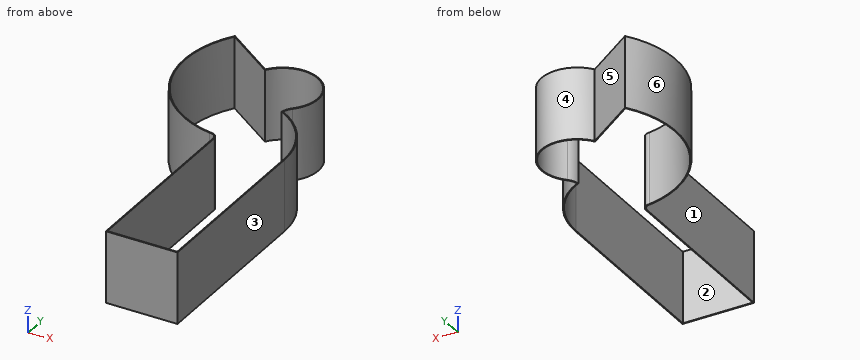
Autodesk Inventor part; units mm, degrees
ref_plane "YZ Plane" through (0, 0, 0) normal (1, 0, 0) x (0, 1, 0)
ref_plane "XZ Plane" through (0, 0, 0) normal (0, 1, 0) x (-1, 0, 0)
ref_plane "XY Plane" through (0, 0, 0) normal (0, 0, 1) x (1, 0, 0)
sketch "Sketch1" plane through (0, 0, 0) normal (0, 0, 1) x (1, 0, 0)
  circle A0 centre (330.2, 1028.7) radius 101.6
  arc A1 (101.3289, 1188.9573) -> (284.1769, 753.1166) centre (330.2, 1028.7) ccw
  circle A2 centre (285.75, 734.1316) radius 19.05
  line L0 (330.2, 1028.7) -> (431.8, 1028.7) construction
  line L1 (0, 1023.3941) -> (50.8, 1023.3941)
  line L2 (50.8, 1023.3941) -> (50.8, 972.5941)
  line L3 (50.8, 972.5941) -> (0, 972.5941)
  line L4 (0, 972.5941) -> (0, 1023.3941)
  line L5 (0, 0) -> (685.8, 0) construction
  line L6 (685.8, 1498.6) -> (0, 1498.6) construction
  line L7 (0, 1498.6) -> (0, 0) construction
  line L8 (304.8, 734.1316) -> (304.8, 213.868)
  line L9 (101.3289, 1188.9573) -> (318.1431, 1498.6) construction
  line L10 (101.3289, 1188.9573) -> (685.8, 1188.9573) construction
  arc A3 (508, 734.1316) -> (260.3446, 954.9248) centre (285.75, 734.1316) ccw
  line L11 (508, 734.1316) -> (508, 213.868)
  line L12 (685.8, 1188.9573) -> (685.8, 0) construction
  line L13 (685.8, 228.9727) -> (685.8, 178.1727)
  line L14 (101.3289, 1188.9573) -> (246.9742, 1086.9754)
  line L15 (304.8, 213.868) -> (508, 213.868)
  arc A4 (401.1312, 955.9585) -> (387.7592, 931.5884) centre (434.38, 921.8609) ccw
  dimension "d0" = 203.2
  dimension "d1" = 279.4
  dimension "d3" = 50.8
  dimension "d4" = 1498.6
  dimension "d5" = 685.8
  dimension "d6" = 38.1
  dimension "d9" = 55
  dimension "d10" = 1028.7
  dimension "d14" = 213.868
  dimension "d20" = 304.8
  dimension "d21" = 177.8
extrude "Extrusion1" add sketch "Sketch1" along normal blind 203.2 contours A0 A3 | A0 A3 L11 L15 L8 A2 A1 L14 | A4 A3 A0 | A3 A0
shell "Shell1" thickness 2.54 removed faces 2 at (372.5333, 560.7104, 0) at (440.2667, 387.2892, 203.2)
properties part number "SketchProfile"
Input: part model. Units: mm. Frame: model coordinates. Face numbers are marked on the shaded views. A direction names the side the tool comes from. Give positions to 0.01 mm unless a question says otherwise; leave off trailing zeros. Order: outer loops, then holes, each group sorted by start corner. A loop starts at its lowest first (then second) coordinate and runs counter-clockwise, first axis right, second up. Notation, with made-up numbers: (-29.75, 12) - (-7.75, 12) arc R26 ccw to (-7.75, 27) - close; hole circle Ø11 at (-29, 88). An arc over 180 degrees is marked (long way). Put each result on its own line as item: value.
Item 1: Access query for the marked faces 1, 2 and 3. Directions: +Z, -Z, +X, -X, +Y, -Y. A direction counts if a zero-diameter tool reaches every point of the face in a straight line with its end or side. Return the directions, or none.
Found:
face 1: +Z, -Z, -X, -Y
face 2: +Z, -Z
face 3: +Z, -Z, +X, +Y, -Y
Item 2: Section query A-A, the plane x = 330.2. Return loops of the section in (y, z), then the cut area to 3 significant figures.
Found:
outline: (213.87, 0) - (216.41, 0) - (216.41, 203.2) - (213.87, 203.2) - close; (1127.76, 0) - (1130.3, 0) - (1130.3, 203.2) - (1127.76, 203.2) - close
area: 1,030 mm^2
Item 3: Section query B-B, the plane y = 1028.7. Return loops of the section in (x, z), then the cut area to 3 significant figures.
Found:
outline: (50.8, 0) - (53.34, 0) - (53.34, 203.2) - (50.8, 203.2) - close; (429.26, 0) - (431.8, 0) - (431.8, 203.2) - (429.26, 203.2) - close
area: 1,030 mm^2
Item 4: Section query C-C, the plane z = 58. Return loops of the section in (x, y), then the cut area to 3 significant figures.
Found:
outline: (101.33, 1188.96) arc R279.4 ccw to (284.18, 753.12) arc R19.05 cw to (304.8, 734.13) - (304.8, 213.87) - (508, 213.87) - (508, 734.13) arc R222.25 ccw to (387.76, 931.59) arc R47.62 cw to (401.13, 955.96) arc R101.6 ccw (long way) to (246.97, 1086.98) - close; hole (101.96, 1185.41) arc R276.86 ccw to (284.29, 755.67) arc R21.59 cw to (307.34, 734.13) - (307.34, 216.41) - (505.46, 216.41) - (505.46, 734.13) arc R219.71 ccw to (384.91, 930.19) arc R50.16 cw to (399.36, 957.78) arc R99.06 ccw (long way) to (247.62, 1083.42) - close
area: 6,650 mm^2
Item 5: Draft query along Y for the marked faces 4, 5 and 6. Return one class per face: +Y half, -Y half, draft (parallel to the pull), parting line (faces both ways), or undercut.
Found:
face 4: undercut
face 5: +Y half
face 6: parting line
Item 6: Ray query, L1, parallel to X at y = 302, z = 72; L2, parallel to X at y = 1028.7, z = 132.5; L3, parallel to Y at x = 122, z = 141. Return the intervals inside material, ascending. Write a range as from..to.
Found:
L1: x = 304.8..307.34, 505.46..508
L2: x = 50.8..53.34, 429.26..431.8
L3: y = 842.37..846.21, 1171.38..1174.48
Item 7: Contact query for flat-ended pins moving along their axis: pin 1 (10 mm diameter, centred on x = 261.5, z = 52.5, fed in from -Y); pin 2 (6 mm diameter, centred on x = 407.5, z = 176.5, fed in from +Y); pin 3 (4 mm diameter, centred on x = 247.5, z = 163.5, fed in from -Y). Output: stop coordinate, or through.
Found:
pin 1: stops at y = 756.66
pin 2: stops at y = 1098
pin 3: stops at y = 761.21
